Can you work these out from the model? Positions are in its coordinate system, mm. Round coordinates to 2 decimals unless told otherwise and drop trailing zeros. Write each loop counter-clockwise with the first axis right and the second up, starting at its lowest first coordinate (ties: lowest second). Pieces come first, ordered by that corner, then holes. Notation, with made-up numbers: (-32, 89) -> (2, 89) arc R10 ccw to (2, 100) -> close; hole circle Ø2 at (16, -38.5). An arc over 180 degrees is marked (long way). Write item = value, one per line. Start each with the question number.
1) I'm going to push a flat-ended pin straight in: pin 1 (3 mm diameter, centred on y = 2, z = 1060, fed in from +X). Where does the tip first touch, or does it pass through?
2) Imagine slicing it at A-A, the plane z = 1330. Please give me the cut outline in (x, y).
3) If I drill on line 1 (X direction, y = -15, z = 1159); line 2 (Y direction, x = 17, z = 1457); line 3 (X direction, y = 16.5, z = 833.5), over which ranges is the centre line in solid material (lowest first)?
from build123d import *

# Parameters (mm, degrees)
BOSS_EXTRUDE1_DEPTH             = 1615
SCHNITT_LINEAR_AUSTRAGEN1_REACH = 1617.619
SKIZZE1_W                       = 10
SKIZZE1_H                       = 10


with BuildPart() as part:
    # Sketch1 → Boss-Extrude1 (new body)
    with BuildSketch(Plane.XY):
        with BuildLine():
            Line((-15.5, -20), (-5, -20))
            Line((-5, -20), (-5, -10))
            Line((-5, -10), (5, -10))
            Line((5, -10), (5, -20))
            Line((5, -20), (15.5, -20))
            ThreePointArc((15.5, -20), (18.681980515, -18.681980515), (20, -15.5))
            Line((20, -15.5), (20, -5))
            Line((20, -5), (10, -5))
            Line((10, -5), (10, 5))
            Line((10, 5), (20, 5))
            Line((20, 5), (20, 15.5))
            ThreePointArc((20, 15.5), (18.681980515, 18.681980515), (15.5, 20))
            Line((15.5, 20), (5, 20))
            Line((5, 20), (5, 10))
            Line((5, 10), (-5, 10))
            Line((-5, 10), (-5, 20))
            Line((-5, 20), (-8, 20))
            Line((-8, 20), (-15, 20))
            Line((-15, 20), (-15.5, 20))
            ThreePointArc((-15.5, 20), (-18.681980515, 18.681980515), (-20, 15.5))
            Line((-20, 15.5), (-20, 5))
            Line((-20, 5), (-10, 5))
            Line((-10, 5), (-10, -5))
            Line((-10, -5), (-20, -5))
            Line((-20, -5), (-20, -15.5))
            ThreePointArc((-20, -15.5), (-18.681980515, -18.681980515), (-15.5, -20))
        make_face()
    extrude(amount=BOSS_EXTRUDE1_DEPTH)

    # Skizze1 → Schnitt-Linear austragen1 (cut, up to next)
    with BuildSketch(Plane(origin=(20, 0, 0), x_dir=(0, 0, -1), z_dir=(1, 0, 0)), mode=Mode.PRIVATE) as schnitt_linear_austragen1_sk1:
        with Locations((-807.5, 15)):
            Rectangle(SKIZZE1_W, SKIZZE1_H)
    schnitt_linear_austragen1_tool1 = extrude(schnitt_linear_austragen1_sk1.sketch, amount=-SCHNITT_LINEAR_AUSTRAGEN1_REACH, mode=Mode.PRIVATE) & part.part
    add(schnitt_linear_austragen1_tool1.solids().sort_by_distance((20, 15, 807.5))[0], mode=Mode.SUBTRACT)


solid = part.part
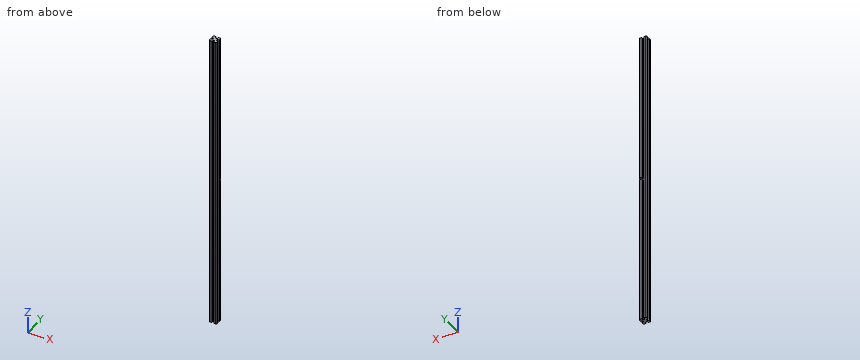
Reported:
q1.pin_1 = 10
q2.outline = (-20, -15.5) arc R4.5 ccw to (-15.5, -20) -> (-5, -20) -> (-5, -10) -> (5, -10) -> (5, -20) -> (15.5, -20) arc R4.5 ccw to (20, -15.5) -> (20, -5) -> (10, -5) -> (10, 5) -> (20, 5) -> (20, 15.5) arc R4.5 ccw to (15.5, 20) -> (5, 20) -> (5, 10) -> (-5, 10) -> (-5, 20) -> (-15.5, 20) arc R4.5 ccw to (-20, 15.5) -> (-20, 5) -> (-10, 5) -> (-10, -5) -> (-20, -5) -> close
q3.line_1 = -20 to -5, 5 to 20
q3.line_2 = -19.74 to -5, 5 to 19.74
q3.line_3 = -19.89 to -5, 5 to 19.89
